```python
from build123d import *

# Parameters (mm, degrees)
SALIENTE_EXTRUIR1_DEPTH = 40
SKETCH2_R               = 4
SKETCH2_R_2             = 2
CUT_EXTRUDE1_DEPTH      = 50
FILLET3_RADIUS          = 20
FILLET3_LENGTH          = 4
CROQUIS3_W              = 40
CROQUIS3_H              = 40
CROQUIS3_R              = 4
CROQUIS3_R_2            = 2
SALIENTE_EXTRUIR2_DEPTH = 4
SALIENTE_EXTRUIR3_START = -4
SKETCH7_W               = 120
SKETCH7_H               = 80
SALIENTE_EXTRUIR3_DEPTH = 24
CROQUIS4_W              = 40
CROQUIS4_H              = 40
CROQUIS4_R              = 4
CROQUIS4_R_2            = 2
SALIENTE_EXTRUIR4_DEPTH = 4
REDONDEO2_RADIUS        = 20
REDONDEO2_LENGTH        = 4
CROQUIS5_R              = 4
CROQUIS5_R_2            = 2
CORTAR_EXTRUIR1_DEPTH   = 50
CROQUIS6_W              = 22.229294361
CROQUIS6_H              = 60
SALIENTE_EXTRUIR5_DEPTH = 4
CROQUIS8_W              = 104
CROQUIS8_H              = 64
CORTAR_EXTRUIR2_DEPTH   = 80
CROQUIS7_W              = 13.68118259
CROQUIS7_H              = 40
SALIENTE_EXTRUIR6_DEPTH = 4
CROQUIS10_W             = 20.658327355
CROQUIS10_H             = 32
SALIENTE_EXTRUIR7_DEPTH = 8


with BuildPart() as part:
    # Croquis2 → Saliente-Extruir1 (new body)
    with BuildSketch(Plane(origin=(0, 0, 0), x_dir=(0, 1, 0), z_dir=(0, 0, 1))):
        Polygon((-16, -6.258064516), (-16, -4.258064516), (-16, 33.741935484), (-20, 33.741935484), (-20, -6.258064516), align=None)
    saliente_extruir1 = extrude(amount=SALIENTE_EXTRUIR1_DEPTH)

    # Sketch2 → Cut-Extrude1 (cut)
    with BuildSketch(Plane.XZ.offset(20)):
        with Locations(Location((-18.741935484, 20, 0), (0, 0, 270))):
            Circle(SKETCH2_R)
        with Locations(Location((-18.741935484, 27, 0), (0, 0, 270))):
            Circle(SKETCH2_R_2)
        with Locations(Location((-11.741935484, 20, 0), (0, 0, 270))):
            Circle(SKETCH2_R_2)
        with Locations(Location((-18.741935484, 13, 0), (0, 0, 270))):
            Circle(SKETCH2_R_2)
        with Locations(Location((-25.741935484, 20, 0), (0, 0, 270))):
            Circle(SKETCH2_R_2)
    extrude(amount=-CUT_EXTRUDE1_DEPTH, mode=Mode.SUBTRACT)

    # Fillet3: full round fillet: the end face becomes a half cylinder, R = half its width
    fillet3_face = Plane((-33.741935484, -18, 20), x_dir=(0, 1, 0), z_dir=(-1, 0, 0))  # on the end face: x along it, z out of the body
    fillet3_slab = fillet3_face.offset(-FILLET3_RADIUS / 2) * Box(FILLET3_LENGTH, 2 * FILLET3_RADIUS, FILLET3_RADIUS, mode=Mode.PRIVATE)  # the body's end, R deep
    fillet3_round = Plane((-13.741935484, -18, 20), x_dir=(-1, 0, 0), z_dir=(0, 1, 0)) * Cylinder(FILLET3_RADIUS, FILLET3_LENGTH, mode=Mode.PRIVATE)  # its axis R under the face
    add(fillet3_slab - fillet3_round, mode=Mode.SUBTRACT)



with BuildPart() as body_2:
    # Croquis3 → Saliente-Extruir2 (new body)
    with BuildSketch(Plane(origin=(0, 0, 20), x_dir=(0, 1, 0), z_dir=(0, 0, 1))):
        with Locations((0, -146.24009387)):
            Rectangle(CROQUIS3_W, CROQUIS3_H)
        with Locations(Location((0, -146.24009387, 0), (0, 0, 270))):
            Circle(CROQUIS3_R, mode=Mode.SUBTRACT)
        with Locations(Location((0, -139.24009387, 0), (0, 0, 270))):
            Circle(CROQUIS3_R_2, mode=Mode.SUBTRACT)
        with Locations(Location((6.662523083, -146.24009387, 0), (0, 0, 270))):
            Circle(CROQUIS3_R_2, mode=Mode.SUBTRACT)
        with Locations(Location((-0.337476917, -153.24009387, 0), (0, 0, 270))):
            Circle(CROQUIS3_R_2, mode=Mode.SUBTRACT)
        with Locations(Location((-7.337476917, -146.24009387, 0), (0, 0, 270))):
            Circle(CROQUIS3_R_2, mode=Mode.SUBTRACT)
    extrude(amount=SALIENTE_EXTRUIR2_DEPTH)


with BuildPart() as part_1:
    add(part.part)

    add(body_2.part)  # Saliente-Extruir3 merges body 2
    # Sketch7 → Saliente-Extruir3 (add)
    with BuildSketch(Plane.XZ.offset(20).offset(SALIENTE_EXTRUIR3_START)):
        with Locations((66.258064516, 40)):
            Rectangle(SKETCH7_W, SKETCH7_H)
    saliente_extruir3 = extrude(amount=SALIENTE_EXTRUIR3_DEPTH)

    # Croquis4 → Saliente-Extruir4 (add)
    with BuildSketch(Plane.XY.offset(80)):
        with Locations((146.039860125, 0)):
            Rectangle(CROQUIS4_W, CROQUIS4_H)
        with Locations((146.039860125, 0)):
            Circle(CROQUIS4_R, mode=Mode.SUBTRACT)
        with Locations((146.039860125, 7)):
            Circle(CROQUIS4_R_2, mode=Mode.SUBTRACT)
        with Locations((153.039860125, -0.581130473)):
            Circle(CROQUIS4_R_2, mode=Mode.SUBTRACT)
        with Locations((146.039860125, -7.581130473)):
            Circle(CROQUIS4_R_2, mode=Mode.SUBTRACT)
        with Locations((139.039860125, -0.581130473)):
            Circle(CROQUIS4_R_2, mode=Mode.SUBTRACT)
    extrude(amount=-SALIENTE_EXTRUIR4_DEPTH)

    # Simetría3: Saliente-Extruir3 across plane
    add(saliente_extruir3.mirror(Plane.ZX))

    # Simetría4: Saliente-Extruir1 across plane
    add(saliente_extruir1.mirror(Plane.ZX))

    # Redondeo2: full round fillet: the end face becomes a half cylinder, R = half its width
    redondeo2_face = Plane((-33.741935484, 18, 20), x_dir=(0, -1, 0), z_dir=(-1, 0, 0))  # on the end face: x along it, z out of the body
    redondeo2_slab = redondeo2_face.offset(-REDONDEO2_RADIUS / 2) * Box(REDONDEO2_LENGTH, 2 * REDONDEO2_RADIUS, REDONDEO2_RADIUS, mode=Mode.PRIVATE)  # the body's end, R deep
    redondeo2_round = Plane((-13.741935484, 18, 20), x_dir=(-1, 0, 0), z_dir=(0, -1, 0)) * Cylinder(REDONDEO2_RADIUS, REDONDEO2_LENGTH, mode=Mode.PRIVATE)  # its axis R under the face
    add(redondeo2_slab - redondeo2_round, mode=Mode.SUBTRACT)

    # Croquis5 → Cortar-Extruir1 (cut)
    with BuildSketch(Plane(origin=(0, 0, 0), x_dir=(-1, 0, 0), z_dir=(0, 1, 0))):
        with Locations(Location((18.741935484, 20, 0), (0, 0, 270))):
            Circle(CROQUIS5_R)
        with Locations(Location((18.741935484, 27, 0), (0, 0, 270))):
            Circle(CROQUIS5_R_2)
        with Locations(Location((25.741935484, 20, 0), (0, 0, 270))):
            Circle(CROQUIS5_R_2)
        with Locations(Location((18.741935484, 13, 0), (0, 0, 270))):
            Circle(CROQUIS5_R_2)
        with Locations(Location((11.741935484, 20, 0), (0, 0, 270))):
            Circle(CROQUIS5_R_2)
    extrude(amount=CORTAR_EXTRUIR1_DEPTH, mode=Mode.SUBTRACT)

    # Croquis6 → Saliente-Extruir5 (add)
    with BuildSketch(Plane.XY.offset(80)):
        with Locations((38.92855935, -10)):
            Rectangle(CROQUIS6_W, CROQUIS6_H)
    extrude(amount=-SALIENTE_EXTRUIR5_DEPTH)

    # Croquis8 → Cortar-Extruir2 (cut)
    with BuildSketch(Plane.XZ.offset(40)):
        with Locations((66.258064516, 40)):
            Rectangle(CROQUIS8_W, CROQUIS8_H)
    extrude(amount=-CORTAR_EXTRUIR2_DEPTH, mode=Mode.SUBTRACT)

    # Croquis7 → Saliente-Extruir6 (add)
    with BuildSketch(Plane(origin=(0, 0, 20), x_dir=(1, 0, 0), z_dir=(0, 0, -1))):
        with Locations((125.098655811, 0)):
            Rectangle(CROQUIS7_W, CROQUIS7_H)
    extrude(amount=-SALIENTE_EXTRUIR6_DEPTH)

    # Croquis10 → Saliente-Extruir7 (add)
    with BuildSketch(Plane.XY.offset(8)):
        with Locations((98.370697006, 0)):
            Rectangle(CROQUIS10_W, CROQUIS10_H)
    extrude(amount=-SALIENTE_EXTRUIR7_DEPTH)


solid = part_1.part
```
Could you check a few things on this model? Use its own coordinates, in mm. A direction names the side the tool comes from. Give positions to 0.01 mm unless a question says otherwise; leave off trailing zeros. Write each loop counter-clockwise with the first axis right and the second up, starting at its lowest first coordinate (ties: lowest second). Pieces come first, ordered by that corner, then holes. Notation, with made-up numbers: (-32.5, 16.25) - (18.5, 16.25) arc R22 cw to (18.5, 30.25) - close; hole circle Ø9 at (-36, 49). An arc over 180 degrees is marked (long way). One line per item, written item: value. Start each with the question number.
Item 1: Which directions (+Z, -Z, +X, -X, +Y, -Y) give clear straight access to the entire face, cutting with the end or side of a thin tool? Please do faces 1 (the face through (149.855, 1.201, 78.028)), 2 (the face through (144.242, 6.75, 21.972)), 3 (the face through (119, -16, 8)), 4 (the face through (14.258, -28, 40)).
Item 2: Imagine slicing it at A-A, the plane x = 63. List the corners of the cut face in (y, z) for me.
Item 3: Imagine slicing it at B-B, the plane z = 57.5. List the corners of the cut face in (x, y) for me, and give its area (3 significant figures).
Item 4: If we mould it in two halves opening along Y, with no side actions, what happens to faces 5 (the face through (137.242, 0.088, 21.972)), 6 (the face through (66, -18, 8)), 7 (the face through (-9.6, -20, 19.7))? For each: +Y half, -Y half, draft (parallel to the pull), parting line (faces both ways), or undercut.
Item 5: I'm going to push flat-ended pins straight in: pin 1 (5 mm diameter, centred on x = -11.74, z = 20, fed in from -Y); pin 2 (20 mm diameter, centred on x = -19.5, z = 30, fed in from +Y); pin 3 (2 mm diameter, centred on y = -5, z = 77.5, fed in from -X); pin 4 (1 mm diameter, centred on x = 103.5, z = 9, fed in from -Y). Where does each tip first touch, or does it pass through?
Item 6: Imagine slicing it at D-D, the plane z = 74. List the corners of the cut face in (x, y) for me, and give its area (3 significant figures).
Item 7: Imagine slicing it at C-C, the plane y = -23.5. List the corners of the cut face in (x, z) for me, and give its area (3 significant figures).
Item 8: Please list where these lines run through material, in increasing order: line 1 (Y direction, x = 14, z = 61); line 2 (Z direction, x = 141, y = 6.5); line 3 (X direction, y = 30, z = 51). Write a range as from..to.
Geometry says:
1. face 1: +Z
1. face 2: -Z
1. face 3: -Z, +X
1. face 4: +Y, -Y
2. outline: (-40, 0) - (-16, 0) - (-16, 8) - (-40, 8) - close; (-40, 72) - (-16, 72) - (-16, 80) - (-40, 80) - close; (16, 0) - (40, 0) - (40, 8) - (16, 8) - close; (16, 72) - (40, 72) - (40, 80) - (16, 80) - close
3. outline: (6.26, -40) - (14.26, -40) - (14.26, -16) - (6.26, -16) - close; (6.26, 16) - (14.26, 16) - (14.26, 40) - (6.26, 40) - close; (118.26, -40) - (126.26, -40) - (126.26, -16) - (118.26, -16) - close; (118.26, 16) - (126.26, 16) - (126.26, 40) - (118.26, 40) - close
3. area: 768 mm^2
4. face 5: undercut
4. face 6: draft
4. face 7: -Y half
5. pin 1: y = -20
5. pin 2: y = 20
5. pin 3: x = 27.81
5. pin 4: through
6. outline: (6.26, -40) - (126.26, -40) - (126.26, -16) - (6.26, -16) - close; (6.26, 16) - (126.26, 16) - (126.26, 40) - (6.26, 40) - close
6. area: 5,760 mm^2
7. outline: (6.26, 0) - (126.26, 0) - (126.26, 80) - (6.26, 80) - close; hole (14.26, 8) - (118.26, 8) - (118.26, 72) - (14.26, 72) - close
7. area: 2,940 mm^2
8. line 1: -40..-16, 16..40
8. line 2: 20..24, 76..80
8. line 3: 6.26..14.26, 118.26..126.26
